Check sheet for the drawn part. Datum: minimum x, y, z corner. Units: mm. A direction names the side the tool comes from. Round coordinates to 2 decimals unless told otherwise and drop trailing zeros. Order: outer loops, then holes, each group sorted by start corner. A loop starts at its lowest first (then second) coordinate and runs counter-clockwise, first axis right, second up. Notation, with made-up numbers: (7, 66.25) -> (63, 66.25) arc R5 cw to (63, 75.25) -> close; hole circle Ø6 at (32, -36). An arc over 180 degrees is marked (long way). Answer in a Markdown table with one row per item.
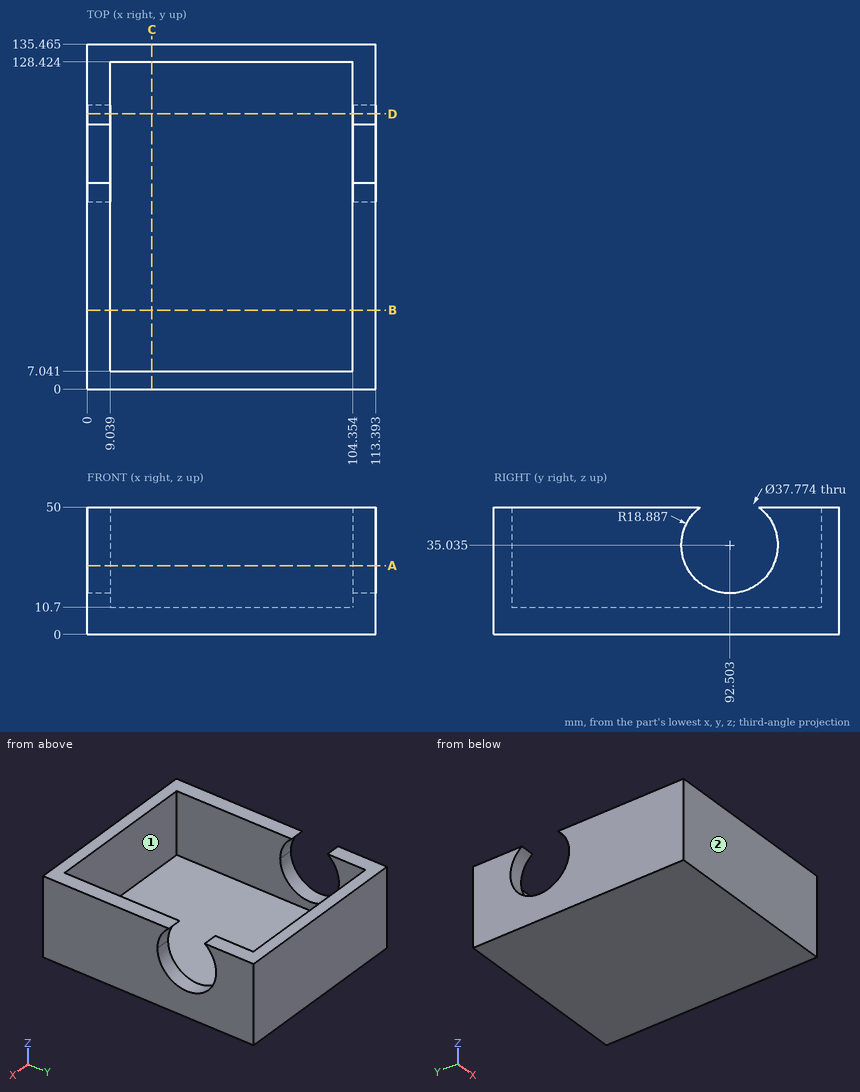
(1) Depth check by flat-ended pin: pin 1 Ø12 at (x, y) = (87.5, 90.5) entering from +Z. Enter the tip coordinate at first touch or a pass-through.
Solutions:
| item | result |
|---|---|
| pin 1 | z = 10.7 |
(2) Section check B-B on y = 31. Record the boundary of the cut face in (x, z) (1 decimal), plus the area to 3 significant figures.
Solutions:
| item | result |
|---|---|
| outline | (0, 0) -> (113.4, 0) -> (113.4, 50) -> (104.4, 50) -> (104.4, 10.7) -> (9, 10.7) -> (9, 50) -> (0, 50) -> close |
| area | 1,920 mm^2 |
(3) Tool access check on the marked faces 1 and 2. Record the directions out of +Z, -Z, +X, -X, +Y, -Y that give a thin tool (end or side, any length) a straight path to the whole face; none if there is none.
Solutions:
| item | result |
|---|---|
| face 1 | +Z |
| face 2 | +Z, -Z, +X, -X, -Y |
(4) Section check C-C on x = 25.5. Record the boundary of the cut face in (y, z) (1 decimal).
Solutions:
| item | result |
|---|---|
| outline | (0, 0) -> (135.5, 0) -> (135.5, 50) -> (128.4, 50) -> (128.4, 10.7) -> (7, 10.7) -> (7, 50) -> (0, 50) -> close |
(5) Section check D-D on y = 108. Record the boundary of the cut face in (x, z) (1 decimal), plus the area to 3 significant figures.
Solutions:
| item | result |
|---|---|
| outline | (0, 0) -> (113.4, 0) -> (113.4, 24.2) -> (104.4, 24.2) -> (104.4, 10.7) -> (9, 10.7) -> (9, 24.2) -> (0, 24.2) -> close; (0, 45.8) -> (9, 45.8) -> (9, 50) -> (0, 50) -> close; (104.4, 45.8) -> (113.4, 45.8) -> (113.4, 50) -> (104.4, 50) -> close |
| area | 1,530 mm^2 |
(6) Section check A-A on z = 27. Record the boundary of the cut face in (x, y) (1 decimal).
Solutions:
| item | result |
|---|---|
| outline | (0, 0) -> (113.4, 0) -> (113.4, 75.4) -> (104.4, 75.4) -> (104.4, 7) -> (9, 7) -> (9, 75.4) -> (0, 75.4) -> close; (0, 109.6) -> (9, 109.6) -> (9, 128.4) -> (104.4, 128.4) -> (104.4, 109.6) -> (113.4, 109.6) -> (113.4, 135.5) -> (0, 135.5) -> close |
(7) Scan lines: probe 1 along Y at (x, z) = (14.5, 15) (1 decimal); probe 2 along X at (y, z) = (12.5, 21) (1 decimal); probe 3 along Z at (x, y) = (14.5, 33.5). Record each from-to range of solid material in increasing order. Write a range as from..to.
Solutions:
| item | result |
|---|---|
| probe 1 | 0..7, 128.4..135.5 |
| probe 2 | 0..9, 104.4..113.4 |
| probe 3 | 0..10.7 |
